Model file for the job. Use its own axes, mm. A direction names the side the tool comes from. Coordinates: 2 decimals unless noted, no trailing zeros. Loops run counter-clockwise (first coordinate to the right, second up) from the corner with the lowest first, then second, coordinate; pieces in that order, holes last. Notation, with made-up numbers: (84, -0.5) -> (95, -0.5) arc R19 ccw to (95, 27.5) -> close; hole circle Ø1 at (-24, -22.5). An arc over 180 degrees is marked (long way). Use one line per item in the form item = value.
```python
from build123d import *

# Parameters (mm, degrees)
SALIENTE_EXTRUIR1_DEPTH   = 2
SALIENTE_EXTRUIR1_2_DEPTH = 2
SALIENTE_EXTRUIR2_DEPTH   = 2
CROQUIS4_R                = 1.5875
CORTAR_EXTRUIR1_DEPTH     = 2


with BuildPart() as part:
    # Croquis2 → Saliente-Extruir1 (new body)
    with BuildSketch(Plane(origin=(0, 19.076482476, 0), x_dir=(1, 0, 0), z_dir=(0, 1, 0))):
        with BuildLine():
            Line((-22.996964511, 5.644085043), (26.003035489, 5.644085043))
            ThreePointArc((26.003035489, 5.644085043), (27.74632721, 3.900793322), (26.003035489, 2.157501601))
            Line((26.003035489, 2.157501601), (-22.996964511, 2.157501601))
            ThreePointArc((-22.996964511, 2.157501601), (-24.740256232, 3.900793322), (-22.996964511, 5.644085043))
        make_face()
    extrude(amount=-SALIENTE_EXTRUIR1_DEPTH)



with BuildPart() as body_2:
    # Croquis2 → Saliente-Extruir1 2 (new body)
    with BuildSketch(Plane(origin=(0, 19.076482476, 0), x_dir=(1, 0, 0), z_dir=(0, 1, 0))):
        with BuildLine():
            Line((-22.996964511, -33.943291721), (26.003035489, -33.943291721))
            ThreePointArc((26.003035489, -33.943291721), (27.74632721, -32.2), (26.003035489, -30.456708279))
            Line((26.003035489, -30.456708279), (-22.996964511, -30.456708279))
            ThreePointArc((-22.996964511, -30.456708279), (-24.740256232, -32.2), (-22.996964511, -33.943291721))
        make_face()
    extrude(amount=-SALIENTE_EXTRUIR1_2_DEPTH)


with BuildPart() as part_1:
    add(part.part)

    add(body_2.part)  # Saliente-Extruir2 merges body 2
    # Croquis3 → Saliente-Extruir2 (add)
    with BuildSketch(Plane(origin=(0, 19.076482476, 0), x_dir=(1, 0, 0), z_dir=(0, 1, 0))):
        with BuildLine():
            ThreePointArc((-24.740256232, 3.900793322), (-24.229657908, 2.668099924), (-22.996964511, 2.157501601))
            Line((-22.996964511, 2.157501601), (26.003035489, 2.157501601))
            ThreePointArc((26.003035489, 2.157501601), (27.235728887, 2.668099924), (27.74632721, 3.900793322))
            ThreePointArc((27.74632721, 3.900793322), (27.235728887, 5.133486719), (26.003035489, 5.644085043))
            Line((26.003035489, 5.644085043), (-22.996964511, 5.644085043))
            ThreePointArc((-22.996964511, 5.644085043), (-24.229657908, 5.133486719), (-24.740256232, 3.900793322))
        make_face()
        with BuildLine():
            Line((26.003035489, 2.157501601), (-22.996964511, 2.157501601))
            ThreePointArc((-22.996964511, 2.157501601), (-24.229657908, 2.668099924), (-24.740256232, 3.900793322))
            Line((-24.740256232, 3.900793322), (-24.740256232, -32.2))
            ThreePointArc((-24.740256232, -32.2), (-24.229657908, -30.967306602), (-22.996964511, -30.456708279))
            Line((-22.996964511, -30.456708279), (26.003035489, -30.456708279))
            ThreePointArc((26.003035489, -30.456708279), (27.235728887, -30.967306602), (27.74632721, -32.2))
            Line((27.74632721, -32.2), (27.74632721, 3.900793322))
            ThreePointArc((27.74632721, 3.900793322), (27.235728887, 2.668099924), (26.003035489, 2.157501601))
        make_face()
        with BuildLine():
            Line((-16.821172495, -18.46), (-16.821172495, -9.84))
            ThreePointArc((-16.821172495, -9.84), (-15.246964511, -8.265792016), (-13.672756527, -9.84))
            Line((-13.672756527, -9.84), (-13.672756527, -18.46))
            ThreePointArc((-13.672756527, -18.46), (-15.246964511, -20.034207984), (-16.821172495, -18.46))
        make_face(mode=Mode.SUBTRACT)
        with BuildLine():
            ThreePointArc((-22.996964511, -30.456708279), (-24.229657908, -30.967306602), (-24.740256232, -32.2))
            ThreePointArc((-24.740256232, -32.2), (-24.229657908, -33.432693398), (-22.996964511, -33.943291721))
            Line((-22.996964511, -33.943291721), (26.003035489, -33.943291721))
            ThreePointArc((26.003035489, -33.943291721), (27.235728887, -33.432693398), (27.74632721, -32.2))
            ThreePointArc((27.74632721, -32.2), (27.235728887, -30.967306602), (26.003035489, -30.456708279))
            Line((26.003035489, -30.456708279), (-22.996964511, -30.456708279))
        make_face()
    extrude(amount=SALIENTE_EXTRUIR2_DEPTH)

    # Croquis4 → Cortar-Extruir1 (cut)
    with BuildSketch(Plane(origin=(0, 21.076482476, 0), x_dir=(1, 0, 0), z_dir=(0, 1, 0))):
        with Locations((-13.784464511, 1.2625)):
            Circle(CROQUIS4_R)
        with Locations((14.790535489, 1.2625)):
            Circle(CROQUIS4_R)
        with Locations((14.790535489, -29.5625)):
            Circle(CROQUIS4_R)
        with Locations((-13.784464511, -29.5625)):
            Circle(CROQUIS4_R)
    extrude(amount=-CORTAR_EXTRUIR1_DEPTH, mode=Mode.SUBTRACT)


solid = part_1.part
```
Q1. Band-saw the part on B-B, the plane x = 21. Write the cut outline in (y, z), and give its area (3 significant figures).
Result:
outline = (17.08, -5.64) -> (21.08, -5.64) -> (21.08, 33.94) -> (17.08, 33.94) -> (17.08, 30.46) -> (19.08, 30.46) -> (19.08, -2.16) -> (17.08, -2.16) -> close
area = 93.1 mm2
Q2. Mould opens along Z. For faces 1 (the face through (-16.821, 20, 14)), 2 (the face through (1, 19, 33.943)), 3 (the face through (2, 18, -2.158)), 4 (the face through (2, 17.076, -4)) say: released by +Z, released by -Z, zero draft, split by the parting line, or undercut.
Result:
face_1 = undercut
face_2 = released by +Z
face_3 = undercut
face_4 = zero draft
Q3. Band-saw the part on A-A, the plane y = 18.45. Write the cut outline in (x, z), and give its area (3 significant figures).
Result:
outline = (-23, -5.64) -> (26, -5.64) arc R1.74 ccw to (26, -2.16) -> (-23, -2.16) arc R1.74 ccw to start; (-23, 30.46) -> (26, 30.46) arc R1.74 ccw to (26, 33.94) -> (-23, 33.94) arc R1.74 ccw to start
area = 361 mm2
Q4. Band-saw the part on C-C, the plane z = 11. Write the cut outline in (x, y), and give its area (3 significant figures).
Result:
outline = (-24.74, 19.08) -> (-16.82, 19.08) -> (-16.82, 21.08) -> (-24.74, 21.08) -> close; (-13.67, 19.08) -> (27.75, 19.08) -> (27.75, 21.08) -> (-13.67, 21.08) -> close
area = 98.7 mm2
Q5. Pin check, flat tips, straight feed: pin 1 Ø2.5 at (x, z) = (-13.78, 29.56) entering from +Y; pin 2 Ø1.5 at (y, z) = (17.5, 10) entering from +X; pin 3 Ø10 at (x, z) = (12, 7) entering from -Y. Stop position of each tip, or through.
Result:
pin_1 = 19.08
pin_2 = through
pin_3 = 19.08
Q6. Band-saw the part on D-D, the plane z = 21. Write the cut outline in (x, y).
Result:
outline = (-24.74, 19.08) -> (27.75, 19.08) -> (27.75, 21.08) -> (-24.74, 21.08) -> close
Q7. Wall check: line 1 along Z through (x, y) = (-18, 18.1); line 2 along X through (y, z) = (19.4, 12.5); line 3 along Z through (x, y) = (-15, 19.95). Give the ranges that are in metal, low to high.
Result:
line_1 = -5.64 to -2.16, 30.46 to 33.94
line_2 = -24.74 to -16.82, -13.67 to 27.75
line_3 = -5.64 to -2.28, -0.24 to 8.29, 20.01 to 28.54, 30.58 to 33.94
Q8. Which spindle directions (+Z, -Z, +X, -X, +Y, -Y) get a long thin tool onto all of the face, cutting with end or side? Do faces 5 (the face through (2, 18, 30.457)), 6 (the face through (-24.622, 18.604, -4.533)), 7 (the face through (-15.212, 20.062, 20.034)), 8 (the face through (13.53, 20.09, 30.53)). Say none if no direction does.
Result:
face_5 = +X, -X, -Y
face_6 = -X, -Y
face_7 = +Y, -Y
face_8 = +Y
